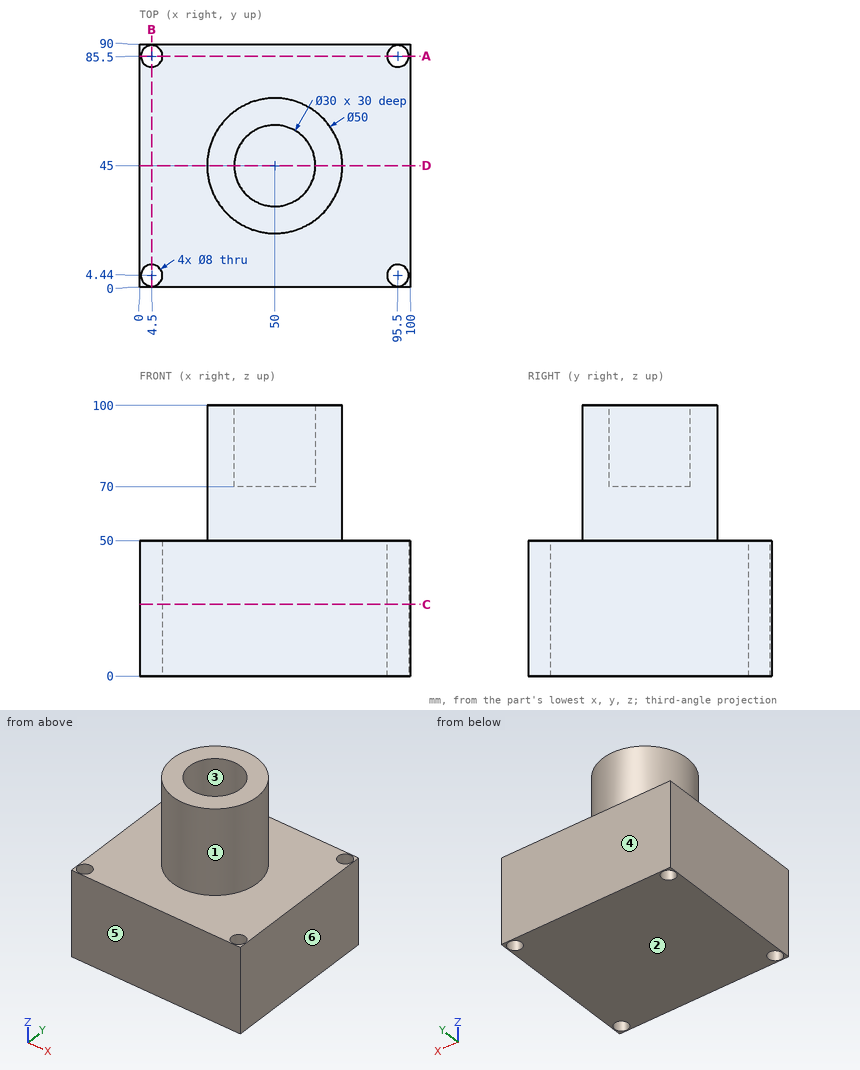
Design review of the part shown in the three views and the two pictorial views. Dimensions are in mm from the part's minimum x, y and z. A direction names the side the tool comes from. Give positions to 0.01 mm unless a question says otherwise; leave off trailing zeros. Loops run counter-clockwise (first coordinate to the right, second up) from the corner with the lowest first, then second, coordinate; pieces in that order, holes last. Notation, with made-up numbers: M -4.5,-25 L 50.5,-25 A11 cw 50.5,-5 Z; hole C 75,65.25 d6. An arc over 180 degrees is marked long. Write item = value, one per line.
Q1. We need section C-C (z = 26.5). Give the boundary of the cut face in (x, y), plus the area to 3 significant figures.
Output values:
outline = M 0,0 L 100,0 L 100,90 L 0,90 Z; hole C 4.5,4.44 d8; hole C 4.5,85.5 d8; hole C 95.5,4.44 d8; hole C 95.5,85.5 d8
area = 8,800 mm^2
Q2. Insertion check: pin 1 (10 mm diameter, centred on y = 70.5, z = 58, fed in from +X); pin 2 (4 mm diameter, centred on x = 28, z = 79.5, fed in from +Y); pin 3 (13 mm diameter, centred on x = 95.5, y = 85.5, fed in from +Z). Each pin has a flat end and moves straight along its axis. Give the tip position at first contact, or say it passes through.
Output values:
pin_1 = 64.31
pin_2 = 60
pin_3 = 50
Q3. To check wall thickness, follow line 1 (X direction, y = 4, z = 25); line 2 (Y direction, x = 95.5, z = 24); line 3 (Y direction, x = 95, z = 12). State the ranges of each line that lie inside material, in increasing order. Write a range as [from, to].
Output values:
line_1 = [0, 0.52], [8.48, 91.52], [99.48, 100]
line_2 = [0, 0.44], [8.44, 81.5], [89.5, 90]
line_3 = [0, 0.47], [8.41, 81.53], [89.47, 90]
Q4. We need section A-A (y = 85.5). Give the boundary of the cut face in (x, z), plus the area to 3 significant figures.
Output values:
outline = M 0,0 L 0.5,0 L 0.5,50 L 0,50 Z; M 8.5,0 L 91.5,0 L 91.5,50 L 8.5,50 Z; M 99.5,0 L 100,0 L 100,50 L 99.5,50 Z
area = 4,200 mm^2
Q5. We need section D-D (y = 45). Give the boundary of the cut face in (x, z).
Output values:
outline = M 0,0 L 100,0 L 100,50 L 75,50 L 75,100 L 65,100 L 65,70 L 35,70 L 35,100 L 25,100 L 25,50 L 0,50 Z
Q6. For the marked faces 1 and 2, list the 3-axis set-ups (+Z, -Z, +X, -X, +Y, -Y) from which the entire face can be reached by the end or side of a thin tool; tool diameter is ignored.
Output values:
face_1 = +Z
face_2 = -Z, +X, -X, +Y, -Y
Q7. Draft analysis for pull direction Y (two halves, no side actions). For the marked faces 3, 4, 5 and 6, state which applies: +Y half, -Y half, draft (parallel to the pull), parting line (faces both ways), or undercut.
Output values:
face_3 = undercut
face_4 = +Y half
face_5 = -Y half
face_6 = draft
Q8. We need section B-B (x = 4.5). Give the boundary of the cut face in (y, z), plus the area to 3 significant figures.
Output values:
outline = M 0,0 L 0.44,0 L 0.44,50 L 0,50 Z; M 8.44,0 L 81.5,0 L 81.5,50 L 8.44,50 Z; M 89.5,0 L 90,0 L 90,50 L 89.5,50 Z
area = 3,700 mm^2
